```python
from build123d import *

# Parameters (mm, degrees)
BRIDA_BASE1_DEPTH            = 1.5875
TALADRO_DE_MARGEN_PARA_M62_D = 6.6


# Sheet-metal steps are written as plain solids
with BuildPart() as part:
    # Croquis1 → Brida base1 (new body)
    with BuildSketch(Plane.XY):
        Polygon((424.28, 230.125), (824.78, -229.645), (-827.22, -229.645), (-827.22, 230.125), align=None)
    extrude(amount=-BRIDA_BASE1_DEPTH)

    # Taladro de margen para M62 (through all)
    with Locations(Plane(origin=(0, 0, -1.5875), x_dir=(-1, 0, 0), z_dir=(0, 0, -1))):
        with Locations((787.22, -209.645), (647.22, -209.645), (507.22, -209.645), (367.22, -209.645), (227.22, -209.645), (87.22, -209.645), (-52.78, -209.645), (-192.78, -209.645), (-332.78, -209.645), (-472.78, -209.645), (-612.78, -209.645), (-752.78, -209.645), (-753.017315716, 208.330699563), (-613.017405979, 208.489676218), (-473.017496241, 208.648652874), (-333.017586504, 208.80762953), (-193.017676767, 208.966606186), (-53.01776703, 209.125582842), (86.982142707, 209.284559498), (226.982052445, 209.443536154), (366.981962182, 209.60251281), (506.981871919, 209.761489466), (646.981781656, 209.920466122), (786.981691393, 210.079442778)):
            Hole(TALADRO_DE_MARGEN_PARA_M62_D / 2)


solid = part.part
```
The model under review builds one solid part; all positions refer to its coordinate system, in mm. Round coordinates to 2 decimals unless told otherwise and drop trailing zeros. Write each loop counter-clockwise with the first axis right and the second up, starting at its lowest first coordinate (ties: lowest second). Pieces come first, ordered by that corner, then holes.
(1) We need section A-A on z = -1.3. Give the number of separate pieces and of enclosed holes in the cut face, and give its area (3 significant figures).
(2) We need section B-B on x = 719. Give the boundary of the cut face in (y, z) (1 decimal).
(3) We need section C-C on y = -41. Give the boundary of the cut face in (x, z).
(4) Wall thickness on L1, parallel to Y at x = 752.78, z = -1.05 (3 decimals); L2, parallel to X at y = -140, z = -1.4; L3, parallel to X at y = -40.5, z = -1.15: over which ranges is each line inside the solid? List them lowest first.
Findings below:
1. separate pieces: 1
1. enclosed holes: 21
1. area: 667,000 mm2
2. outline: (-229.6, -1.6) - (-108.2, -1.6) - (-108.2, 0) - (-229.6, 0) - close
3. outline: (-827.22, -1.59) - (660.45, -1.59) - (660.45, 0) - (-827.22, 0) - close
4. L1: y = -229.645 to -212.945, -206.345 to -146.99
4. L2: x = -827.22 to 746.69
4. L3: x = -827.22 to 660.02
